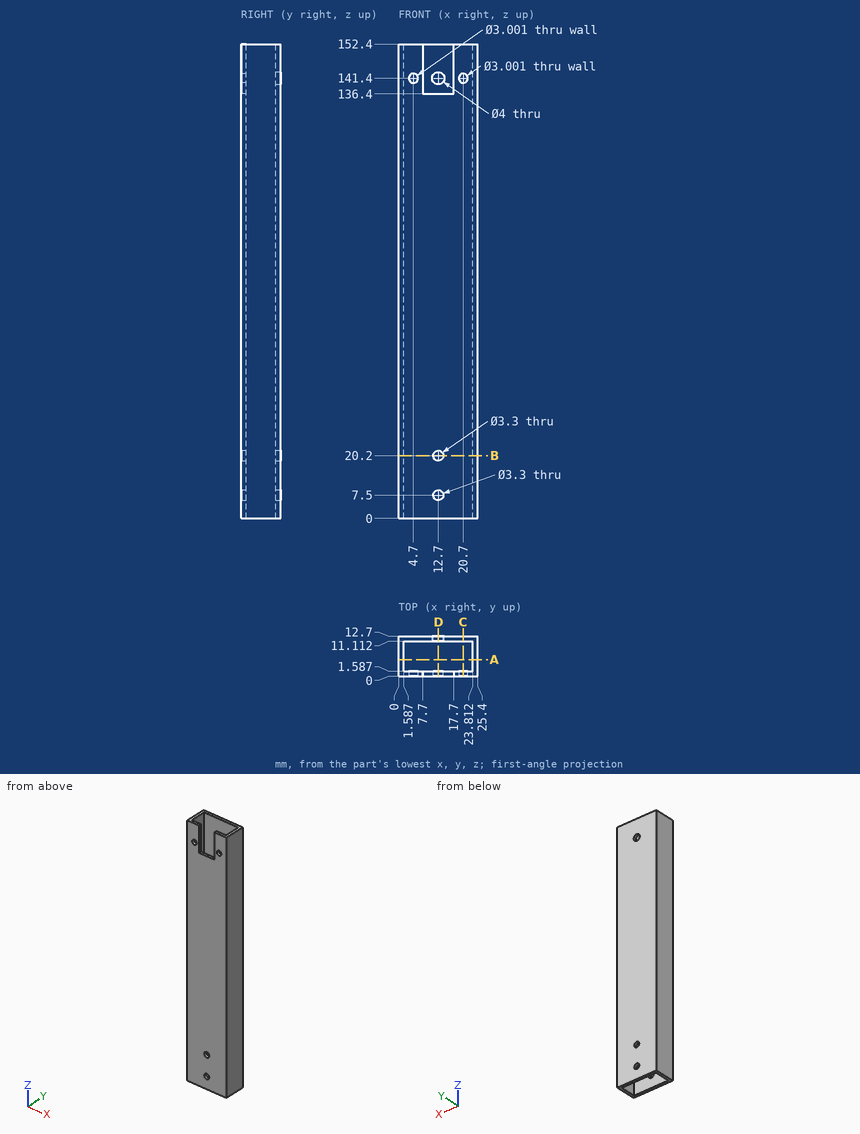
Answer from the drawing. Dimensions are ordinates in mm from the lowest x, y and z of the part. Round coordinates to 2 decimals unless told otherwise and drop trailing zeros. Loops run counter-clockwise (first coordinate to the right, second up) from the corner with the lowest first, then second, coordinate; pieces in that order, holes last.
Q1. Consider probe 1 along Z at (x, y) = (12.7, 0.35); probe 2 along X at (y, z) = (7, 93.5); probe 3 along Y at (x, z) = (16.5, 59.5). Determine where each line is inside the solid, lowest interval first.
Q2. Section D-D on x = 12.7 is taken. Write down the section's boundary in (y, z).
Q3. Section C-C on x = 20.7 is taken. Write down the section's boundary in (y, z).
Q4. Each of these flat-tipped pins is pushed along its axis until it touches: pin 1 (0.8 mm diameter, centred on x = 14.5, y = 1, fed in from +Z); pin 2 (2.5 mm diameter, centred on x = 4.7, z = 141.4, fed in from -Y). Where does it stop, or does it pass through?
Q5. Section B-B on z = 20.2 is taken. Write down the section's boundary in (x, y).
Q6. Section A-A on y = 5.25 is taken. Write down the section's boundary in (x, z).
Output:
1. probe 1: z = 0 to 5.85, 9.15 to 18.55, 21.85 to 136.4
1. probe 2: x = 0 to 1.59, 23.81 to 25.4
1. probe 3: y = 0 to 1.59, 11.11 to 12.7
2. outline: (0, 0) - (1.59, 0) - (1.59, 5.85) - (0, 5.85) - close; (0, 9.15) - (1.59, 9.15) - (1.59, 18.55) - (0, 18.55) - close; (0, 21.85) - (1.59, 21.85) - (1.59, 136.4) - (0, 136.4) - close; (11.11, 0) - (12.7, 0) - (12.7, 5.85) - (11.11, 5.85) - close; (11.11, 9.15) - (12.7, 9.15) - (12.7, 18.55) - (11.11, 18.55) - close; (11.11, 21.85) - (12.7, 21.85) - (12.7, 139.4) - (11.11, 139.4) - close; (11.11, 143.4) - (12.7, 143.4) - (12.7, 152.4) - (11.11, 152.4) - close
3. outline: (0, 0) - (1.59, 0) - (1.59, 139.9) - (0, 139.9) - close; (0, 142.9) - (1.59, 142.9) - (1.59, 152.4) - (0, 152.4) - close; (11.11, 0) - (12.7, 0) - (12.7, 152.4) - (11.11, 152.4) - close
4. pin 1: stops at z = 136.4
4. pin 2: stops at y = 11.11
5. outline: (0, 0) - (11.05, 0) - (11.05, 1.59) - (1.59, 1.59) - (1.59, 11.11) - (11.05, 11.11) - (11.05, 12.7) - (0, 12.7) - close; (14.35, 0) - (25.4, 0) - (25.4, 12.7) - (14.35, 12.7) - (14.35, 11.11) - (23.81, 11.11) - (23.81, 1.59) - (14.35, 1.59) - close
6. outline: (0, 0) - (1.59, 0) - (1.59, 152.4) - (0, 152.4) - close; (23.81, 0) - (25.4, 0) - (25.4, 152.4) - (23.81, 152.4) - close
